```python
from build123d import *

# Parameters (mm, degrees)
SKETCH2_R                  = 13.6779
CUT_EXTRUDE1_DEPTH         = 45.010218722
F_4_40_TAPPED_HOLE2_REACH  = 46.01
F_4_40_TAPPED_HOLE2_BORE_R = 1.1303
CIRPATTERN1_COUNT          = 3
F_4_40_TAPPED_HOLE3_REACH  = 46.01
F_4_40_TAPPED_HOLE3_BORE_R = 1.1303
CIRPATTERN2_COUNT          = 3


with BuildPart() as part:
    # Sketch1 → Revolve1 (revolve)
    with BuildSketch(Plane.XY, mode=Mode.PRIVATE) as revolve1_sk:
        Polygon((4.826, 20.574), (4.826, 14.605), (7.2136, 14.605), (7.2136, 20.574), (7.8232, 20.574), (7.8232, 14.605), (10.2108, 14.605), (10.2108, 20.574), (10.8204, 20.574), (10.8204, 14.605), (13.208, 14.605), (13.208, 20.574), (13.8176, 20.574), (13.8176, 14.605), (16.2052, 14.605), (16.2052, 20.574), (16.8148, 20.574), (16.8148, 14.605), (19.2024, 14.605), (19.2024, 20.574), (19.812, 20.574), (19.812, 14.605), (22.1996, 14.605), (22.1996, 20.574), (22.8092, 20.574), (22.8092, 14.605), (25.1968, 14.605), (25.1968, 20.574), (25.8064, 20.574), (25.8064, 14.605), (28.194, 14.605), (28.194, 20.574), (33.02, 20.574), (33.02, 0), (0, 0), (0, 20.574), align=None)
    revolve(revolve1_sk.sketch.rotate(Axis((0, 0, 0), (1, 0, 0)), 90), axis=Axis((0, 0, 0), (1, 0, 0)))

    # Sketch2 → Cut-Extrude1 (cut, through all)
    with BuildSketch(Plane.ZY):
        Circle(SKETCH2_R)
    extrude(amount=-CUT_EXTRUDE1_DEPTH, mode=Mode.SUBTRACT)

    # #4-40 Tapped Hole2 bore → #4-40 Tapped Hole2 (cut, up to next)
    with BuildSketch(Plane.ZY, mode=Mode.PRIVATE) as f_4_40_tapped_hole2_sk1:
        with Locations((0, 17.0688)):
            Circle(F_4_40_TAPPED_HOLE2_BORE_R)
    f_4_40_tapped_hole2_tool1 = extrude(f_4_40_tapped_hole2_sk1.sketch, amount=-F_4_40_TAPPED_HOLE2_REACH, mode=Mode.PRIVATE) & part.part
    f_4_40_tapped_hole2 = f_4_40_tapped_hole2_tool1.solids().sort_by_distance((0, 17.0688, 0))[0]
    add(f_4_40_tapped_hole2, mode=Mode.SUBTRACT)

    # CirPattern1: #4-40 Tapped Hole2 ×3 about axis
    cirpattern1_axis = Axis((0, 0, 0), (1, 0, 0))
    for i in range(1, CIRPATTERN1_COUNT):
        add(f_4_40_tapped_hole2.rotate(cirpattern1_axis, i * 360 / CIRPATTERN1_COUNT), mode=Mode.SUBTRACT)

    # #4-40 Tapped Hole3 bore → #4-40 Tapped Hole3 (cut, up to next)
    with BuildSketch(Plane(origin=(33.02, 0, 0), x_dir=(0, 0, -1), z_dir=(1, 0, 0)), mode=Mode.PRIVATE) as f_4_40_tapped_hole3_sk1:
        with Locations((0, 17.0688)):
            Circle(F_4_40_TAPPED_HOLE3_BORE_R)
    f_4_40_tapped_hole3_tool1 = extrude(f_4_40_tapped_hole3_sk1.sketch, amount=-F_4_40_TAPPED_HOLE3_REACH, mode=Mode.PRIVATE) & part.part
    f_4_40_tapped_hole3 = f_4_40_tapped_hole3_tool1.solids().sort_by_distance((33.02, 17.0688, 0))[0]
    add(f_4_40_tapped_hole3, mode=Mode.SUBTRACT)

    # CirPattern2: #4-40 Tapped Hole3 ×3 about axis
    cirpattern2_axis = Axis((0, 0, 0), (1, 0, 0))
    for i in range(1, CIRPATTERN2_COUNT):
        add(f_4_40_tapped_hole3.rotate(cirpattern2_axis, i * 360 / CIRPATTERN2_COUNT), mode=Mode.SUBTRACT)


solid = part.part
```
Input: part model. Units: mm. Frame: model coordinates. A direction names the side the tool comes from. Give positions to 0.01 mm unless a question says otherwise; leave off trailing zeros. Order: outer loops, then holes, each group sorted by start corner. A loop starts at its lowest first (then second) coordinate and runs counter-clockwise, first axis right, second up. Notation, with made-up numbers: (5.5, -30) - (61.5, -30) arc R18 ccw to (61.5, -5) - close; hole circle Ø4 at (44.25, 44.25). An arc over 180 degrees is marked (long way). Use a Markdown table: item, result.
(1) Line query: line 1 (Z direction, x = 20, y = 9); line 2 (Z direction, x = 25.5, y = 7.5); line 3 (Y direction, x = 4, z = 8). Output: solid intervals per line, ascending. Write a range as from..to.
Computed values:
| item | result |
|---|---|
| line 1 | z = -11.5..-10.3, 10.3..11.5 |
| line 2 | z = -19.16..-11.44, 11.44..19.16 |
| line 3 | y = -18.95..-11.09, 11.09..18.95 |
(2) Access query for faces 1 (the cylindrical face through (7.52, -20.4, -2.68)), 2 (the flat face through (25.197, -14, 5)), 3 (the cylindrical face through (30.64, -8.97, 13.74)). Directions: +Z, -Z, +X, -X, +Y, -Y. A direction counts if a zero-diameter tool reaches every point of the face in a straight line with its end or side. Return the directions, or none.
Computed values:
| item | result |
|---|---|
| face 1 | +X, -X |
| face 2 | none |
| face 3 | +X |
(3) Section query A-A (z = 0). State how many separate pieces and enclosed holes the cut face has, then the cut area to 3 significant figures.
Computed values:
| item | result |
|---|---|
| separate pieces | 4 |
| enclosed holes | 0 |
| area | 206 mm2 |
(4) Draft query along Y for faces 4 (the cylindrical face through (2.379, 15.965, -0.245)), 5 (the cylindrical face through (12.03, -14.48, -1.9)), 6 (the cylindrical face through (30.641, 15.965, 0.245)), 7 (the flat face through (22.809, -14, -5)). Return one class per face: released by +Y, released by -Y, zero draft, split by the parting line, or undercut.
Computed values:
| item | result |
|---|---|
| face 4 | undercut |
| face 5 | split by the parting line |
| face 6 | undercut |
| face 7 | zero draft |
(5) Section query B-B (x = 8.5). Output: boundary loops of the cut face in (y, z) (3 decimals), then the cut area to 3 significant figures.
Computed values:
| item | result |
|---|---|
| outline | circle Ø29.21 at (0, 0); hole circle Ø27.356 at (0, 0) |
| area | 82.4 mm2 |
(6) Pin query (flat end, axial travel): pin 1 (12 mm diameter, centred on y = 4.5, z = 7.5, fed in from -X); pin 2 (1.8 mm diameter, centred on y = 17.07, z = 0, fed in from +X); pin 3 (10 mm diameter, centred on x = 22.5, y = 11.5, fed in from -Z); pin 4 (1 mm diameter, centred on x = 17.5, y = -13.5, fed in from -Z). Return the tip coordinate at first contact, or that it passes through.
Computed values:
| item | result |
|---|---|
| pin 1 | stops at x = 0 |
| pin 2 | stops at x = 25.81 |
| pin 3 | stops at z = -19.52 |
| pin 4 | stops at z = -6.66 |
